Model file for the job. Use its own axes, mm. Coordinates: 2 decimals unless noted, no trailing zeros. Write each loop counter-clockwise with the first axis right and the second up, starting at its lowest first coordinate (ties: lowest second). Pieces come first, ordered by that corner, then holes. Notation, with made-up numbers: M 21.5,73 L 26.5,73 A15 ccw 26.5,91 Z; hole C 74,45 d3. An arc over 180 degrees is marked long. One line per question, with ' | ' between items. Start each with the question number.
(1) Flat gauge pin, fed straight in: pin 1 Ø9 at (x, z) = (-0.33, 0.13) entering from -Y. Where does the tip first touch, or does it go through?
(2) Cut at B-B (z = -41.5). Write the cut outline in (x, y), plus the area to 3 significant figures.
(3) Cut at C-C (y = -1.9). Count the separate pieces of the cut face and the enclosed holes in it, plus the area to 3 significant figures.
(4) Cut at A-A (x = 2). Write the cut outline in (y, z), plus the area to 3 significant figures.
(5) Wall check: probe 1 along X at (y, z) = (-2.6, -14); probe 2 along X at (y, z) = (-2.1, -58.5); probe 3 along Z at (x, y) = (22.5, -2.6). Give the ranges that are in metal, low to high.
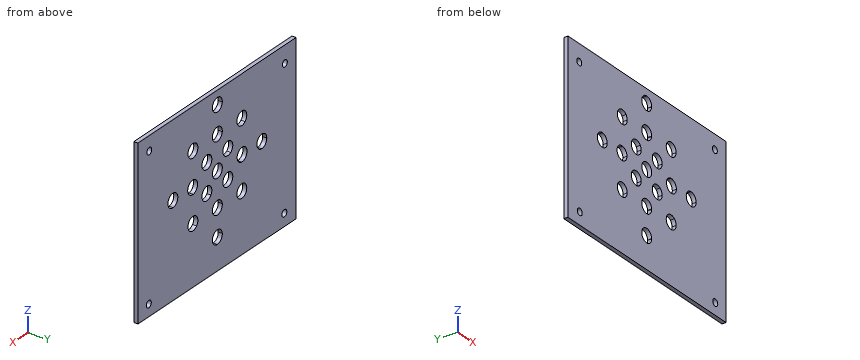
from build123d import *

# Parameters (mm, degrees)
F0_R     = 2.5
F0_R_2   = 5
F1_DEPTH = 3


with BuildPart() as f1:
    # F0 (on Front) → F1 (new body)
    with BuildSketch(Plane.XZ):
        Polygon((0, -68), (80, -68), (80, 55), (-80, 55.240198642), (-80, -68), align=None)
        with Locations((-68.1081116199, -58.9685998857)):
            Circle(F0_R, mode=Mode.SUBTRACT)
        with Locations((69.0506994724, -59.3423657119)):
            Circle(F0_R, mode=Mode.SUBTRACT)
        Polygon((49.6701618657, 0.1303526806), (49.6701618657, -49.8696473194), (-0.3298381532, -49.8696473194), (-50.3298381343, -49.8696473194), (-50.3298381343, 0.130352625), (-50.3298381343, 50.1303526806), (-0.3298380849, 50.1303526806), (49.6701618657, 50.1303526806), align=None, mode=Mode.SUBTRACT)
        with Locations((-68.6089098454, 42.6927655935)):
            Circle(F0_R, mode=Mode.SUBTRACT)
        with Locations((68.6089023948, 44.4455519319)):
            Circle(F0_R, mode=Mode.SUBTRACT)
        with BuildLine():
            ThreePointArc((-45.0520603566, -4.8619253071), (-32.1496432877, -31.6894524728), (-5.322116122, -44.5918695417))
            ThreePointArc((-5.322116122, -44.5918695417), (-0.3298381343, -39.8696473194), (4.6624398533, -44.5918695417))
            ThreePointArc((4.6624398533, -44.5918695417), (31.489967019, -31.6894524728), (44.3923840879, -4.8619253071))
            ThreePointArc((44.3923840879, -4.8619253071), (39.6701618657, 0.1303526806), (44.3923840879, 5.1226306682))
            ThreePointArc((44.3923840879, 5.1226306682), (31.489967019, 31.950157834), (4.6624398533, 44.8525749028))
            ThreePointArc((4.6624398533, 44.8525749028), (-0.3298381343, 40.1303526806), (-5.322116122, 44.8525749028))
            ThreePointArc((-5.322116122, 44.8525749028), (-32.1496432877, 31.950157834), (-45.0520603566, 5.1226306682))
            ThreePointArc((-45.0520603566, 5.1226306682), (-41.6974223481, 3.5662740353), (-40.3298381343, 0.1303526806))
            ThreePointArc((-40.3298381343, 0.1303526806), (-41.6974223481, -3.3055686741), (-45.0520603566, -4.8619253071))
        make_face()
        with BuildLine():
            ThreePointArc((27.6928642243, 21.1000487327), (32.8800593553, 11.1803621251), (34.6701618657, 0.1303526806))
            ThreePointArc((34.6701618657, 0.1303526806), (32.8800593553, -10.9196567639), (27.6928642243, -20.8393433716))
            ThreePointArc((27.6928642243, -20.8393433716), (28.9669661089, -22.5411058021), (29.4188992072, -24.618384661))
            ThreePointArc((29.4188992072, -24.618384661), (26.1660101872, -29.303211576), (20.6398579178, -27.8923496781))
            ThreePointArc((20.6398579178, -27.8923496781), (-0.3298381343, -34.8696473194), (-21.2995341865, -27.8923496781))
            ThreePointArc((-21.2995341865, -27.8923496781), (-28.6141093818, -28.1539185669), (-28.352540493, -20.8393433716))
            ThreePointArc((-28.352540493, -20.8393433716), (-35.3298381343, 0.1303526806), (-28.352540493, 21.1000487327))
            ThreePointArc((-28.352540493, 21.1000487327), (-28.6141093818, 28.414623928), (-21.2995341865, 28.1530550392))
            ThreePointArc((-21.2995341865, 28.1530550392), (-0.3298381343, 35.1303526806), (20.6398579178, 28.1530550392))
            ThreePointArc((20.6398579178, 28.1530550392), (26.1660101872, 29.5639169371), (29.4188992072, 24.8790900221))
            ThreePointArc((29.4188992072, 24.8790900221), (28.9669661089, 22.8018111633), (27.6928642243, 21.1000487327))
        make_face(mode=Mode.SUBTRACT)
        with BuildLine():
            ThreePointArc((27.6928642243, -20.8393433716), (32.8800593553, -10.9196567639), (34.6701618657, 0.1303526806))
            ThreePointArc((34.6701618657, 0.1303526806), (32.8800593553, 11.1803621251), (27.6928642243, 21.1000487327))
            ThreePointArc((27.6928642243, 21.1000487327), (20.8833653012, 21.3435561162), (20.6398579178, 28.1530550392))
            ThreePointArc((20.6398579178, 28.1530550392), (-0.3298381343, 35.1303526806), (-21.2995341865, 28.1530550392))
            ThreePointArc((-21.2995341865, 28.1530550392), (-20.3937485609, 26.6262010021), (-20.0785754759, 24.8790900221))
            ThreePointArc((-20.0785754759, 24.8790900221), (-23.0012966171, 20.3310231204), (-28.352540493, 21.1000487327))
            ThreePointArc((-28.352540493, 21.1000487327), (-35.3298381343, 0.1303526806), (-28.352540493, -20.8393433716))
            ThreePointArc((-28.352540493, -20.8393433716), (-23.0012966171, -20.0703177592), (-20.0785754759, -24.618384661))
            ThreePointArc((-20.0785754759, -24.618384661), (-20.3937485609, -26.365495641), (-21.2995341865, -27.8923496781))
            ThreePointArc((-21.2995341865, -27.8923496781), (-0.3298381343, -34.8696473194), (20.6398579178, -27.8923496781))
            ThreePointArc((20.6398579178, -27.8923496781), (20.8833653012, -21.082850755), (27.6928642243, -20.8393433716))
        make_face()
        with BuildLine():
            ThreePointArc((4.6450990512, 24.6303526806), (17.3478313953, 17.8080222102), (24.1701618657, 5.1052898661))
            ThreePointArc((24.1701618657, 5.1052898661), (28.0242638319, 3.8384519241), (29.6701618657, 0.1303526806))
            ThreePointArc((29.6701618657, 0.1303526806), (28.0242638319, -3.577746563), (24.1701618657, -4.844584505))
            ThreePointArc((24.1701618657, -4.844584505), (17.3478313953, -17.5473168491), (4.6450990512, -24.3696473194))
            ThreePointArc((4.6450990512, -24.3696473194), (4.6638922312, -24.6193334441), (4.6701618657, -24.8696473194))
            ThreePointArc((4.6701618657, -24.8696473194), (-0.5801520096, -29.863377685), (-5.3047753199, -24.3696473194))
            ThreePointArc((-5.3047753199, -24.3696473194), (-18.007507664, -17.5473168491), (-24.8298381343, -4.844584505))
            ThreePointArc((-24.8298381343, -4.844584505), (-30.3298381343, 0.1303526806), (-24.8298381343, 5.1052898661))
            ThreePointArc((-24.8298381343, 5.1052898661), (-18.007507664, 17.8080222102), (-5.3047753199, 24.6303526806))
            ThreePointArc((-5.3047753199, 24.6303526806), (-0.5801520096, 30.1240830461), (4.6701618657, 25.1303526806))
            ThreePointArc((4.6701618657, 25.1303526806), (4.6638922312, 24.8800388053), (4.6450990512, 24.6303526806))
        make_face(mode=Mode.SUBTRACT)
        with BuildLine():
            ThreePointArc((24.1701618657, -4.844584505), (19.6701618657, 0.1303526806), (24.1701618657, 5.1052898661))
            ThreePointArc((24.1701618657, 5.1052898661), (17.3478313953, 17.8080222102), (4.6450990512, 24.6303526806))
            ThreePointArc((4.6450990512, 24.6303526806), (-0.3298381343, 20.1303526806), (-5.3047753199, 24.6303526806))
            ThreePointArc((-5.3047753199, 24.6303526806), (-18.007507664, 17.8080222102), (-24.8298381343, 5.1052898661))
            ThreePointArc((-24.8298381343, 5.1052898661), (-21.6217388908, 3.4844546468), (-20.3298381343, 0.1303526806))
            ThreePointArc((-20.3298381343, 0.1303526806), (-21.6217388908, -3.2237492857), (-24.8298381343, -4.844584505))
            ThreePointArc((-24.8298381343, -4.844584505), (-18.007507664, -17.5473168491), (-5.3047753199, -24.3696473194))
            ThreePointArc((-5.3047753199, -24.3696473194), (-0.3298381343, -19.8696473194), (4.6450990512, -24.3696473194))
            ThreePointArc((4.6450990512, -24.3696473194), (17.3478313953, -17.5473168491), (24.1701618657, -4.844584505))
        make_face()
        with BuildLine():
            ThreePointArc((13.1735913764, 6.6616153035), (14.2912330073, 3.4806181431), (14.6701618657, 0.1303526806))
            ThreePointArc((14.6701618657, 0.1303526806), (14.2912330073, -3.219912782), (13.1735913764, -6.4009099423))
            ThreePointArc((13.1735913764, -6.4009099423), (14.7199684496, -8.1832312619), (15.2767635834, -10.4762490372))
            ThreePointArc((15.2767635834, -10.4762490372), (11.7971754562, -15.2394777465), (6.2014244886, -13.3730768301))
            ThreePointArc((6.2014244886, -13.3730768301), (-0.3298381343, -14.8696473194), (-6.8611007573, -13.3730768301))
            ThreePointArc((-6.8611007573, -13.3730768301), (-14.4719737581, -14.0117829432), (-13.833267645, -6.4009099423))
            ThreePointArc((-13.833267645, -6.4009099423), (-15.3298381343, 0.1303526806), (-13.833267645, 6.6616153035))
            ThreePointArc((-13.833267645, 6.6616153035), (-14.4719737581, 14.2724883043), (-6.8611007573, 13.6337821913))
            ThreePointArc((-6.8611007573, 13.6337821913), (-0.3298381343, 15.1303526806), (6.2014244886, 13.6337821913))
            ThreePointArc((6.2014244886, 13.6337821913), (11.7971754562, 15.5001831077), (15.2767635834, 10.7369543984))
            ThreePointArc((15.2767635834, 10.7369543984), (14.7199684496, 8.4439366231), (13.1735913764, 6.6616153035))
        make_face(mode=Mode.SUBTRACT)
        with BuildLine():
            Line((-0.3298381532, -49.8696473194), (49.6701618657, -49.8696473194))
            Line((49.6701618657, -49.8696473194), (49.6701618657, 0.1303526806))
            ThreePointArc((49.6701618657, 0.1303526806), (48.1060832203, -3.5020631057), (44.3923840879, -4.8619253071))
            ThreePointArc((44.3923840879, -4.8619253071), (31.489967019, -31.6894524728), (4.6624398533, -44.5918695417))
            ThreePointArc((4.6624398533, -44.5918695417), (4.6682309897, -44.7307047744), (4.6701618657, -44.8696473194))
            ThreePointArc((4.6701618657, -44.8696473194), (3.2056957649, -48.405181232), (-0.3298381532, -49.8696473194))
        make_face()
        with BuildLine():
            Line((-50.3298381343, -49.8696473194), (-0.3298381532, -49.8696473194))
            ThreePointArc((-0.3298381532, -49.8696473194), (-3.9622539271, -48.3055686673), (-5.322116122, -44.5918695417))
            ThreePointArc((-5.322116122, -44.5918695417), (-32.1496432877, -31.6894524728), (-45.0520603566, -4.8619253071))
            ThreePointArc((-45.0520603566, -4.8619253071), (-48.7657594688, -3.5020631248), (-50.3298381343, 0.130352625))
            Line((-50.3298381343, 0.130352625), (-50.3298381343, -49.8696473194))
        make_face()
        with BuildLine():
            ThreePointArc((44.3923840879, 5.1226306682), (48.1060832203, 3.7627684669), (49.6701618657, 0.1303526806))
            Line((49.6701618657, 0.1303526806), (49.6701618657, 50.1303526806))
            Line((49.6701618657, 50.1303526806), (-0.3298380849, 50.1303526806))
            ThreePointArc((-0.3298380849, 50.1303526806), (3.205695789, 48.665886569), (4.6701618657, 45.1303526806))
            ThreePointArc((4.6701618657, 45.1303526806), (4.6682309897, 44.9914101355), (4.6624398533, 44.8525749028))
            ThreePointArc((4.6624398533, 44.8525749028), (31.489967019, 31.950157834), (44.3923840879, 5.1226306682))
        make_face()
        with BuildLine():
            Line((-50.3298381343, 50.1303526806), (-50.3298381343, 0.130352625))
            ThreePointArc((-50.3298381343, 0.130352625), (-48.7657595092, 3.7627684478), (-45.0520603566, 5.1226306682))
            ThreePointArc((-45.0520603566, 5.1226306682), (-32.1496432877, 31.950157834), (-5.322116122, 44.8525749028))
            ThreePointArc((-5.322116122, 44.8525749028), (-3.9622539037, 48.5662740532), (-0.3298380849, 50.1303526806))
            Line((-0.3298380849, 50.1303526806), (-50.3298381343, 50.1303526806))
        make_face()
        with BuildLine():
            ThreePointArc((13.1735913764, -6.4009099423), (14.2912330073, -3.219912782), (14.6701618657, 0.1303526806))
            ThreePointArc((14.6701618657, 0.1303526806), (14.2912330073, 3.4806181431), (13.1735913764, 6.6616153035))
            ThreePointArc((13.1735913764, 6.6616153035), (6.7412296775, 7.2014204924), (6.2014244886, 13.6337821913))
            ThreePointArc((6.2014244886, 13.6337821913), (-0.3298381343, 15.1303526806), (-6.8611007573, 13.6337821913))
            ThreePointArc((-6.8611007573, 13.6337821913), (-6.1732111428, 12.2573662711), (-5.9364398521, 10.7369543984))
            ThreePointArc((-5.9364398521, 10.7369543984), (-8.6434220769, 6.2937495323), (-13.833267645, 6.6616153035))
            ThreePointArc((-13.833267645, 6.6616153035), (-15.3298381343, 0.1303526806), (-13.833267645, -6.4009099423))
            ThreePointArc((-13.833267645, -6.4009099423), (-8.6434220769, -6.0330441711), (-5.9364398521, -10.4762490372))
            ThreePointArc((-5.9364398521, -10.4762490372), (-6.1732111428, -11.99666091), (-6.8611007573, -13.3730768301))
            ThreePointArc((-6.8611007573, -13.3730768301), (-0.3298381343, -14.8696473194), (6.2014244886, -13.3730768301))
            ThreePointArc((6.2014244886, -13.3730768301), (6.7412296775, -6.9407151313), (13.1735913764, -6.4009099423))
        make_face()
        with Locations((-0.3298381343, 0.1303526806)):
            Circle(F0_R_2, mode=Mode.SUBTRACT)
    extrude(amount=F1_DEPTH)


solid = f1.part
Filled in:
1) pin 1: through
2) outline: M -80,-3 L -4.02,-3 L -4.02,0 L -80,0 Z; M 3.36,-3 L 80,-3 L 80,0 L 3.36,0 Z | area: 458 mm²
3) separate pieces: 1 | enclosed holes: 21 | area: 18,300 mm²
4) outline: M -3,-68 L 0,-68 L 0,-49.29 L -3,-49.29 Z; M -3,-40.45 L 0,-40.45 L 0,-29.29 L -3,-29.29 Z; M -3,-20.45 L 0,-20.45 L 0,-4.29 L -3,-4.29 Z; M -3,4.55 L 0,4.55 L 0,20.71 L -3,20.71 Z; M -3,29.55 L 0,29.55 L 0,40.71 L -3,40.71 Z; M -3,49.55 L 0,49.55 L 0,55.12 L -3,55.12 Z | area: 237 mm²
5) probe 1: -80 to -14.48, -7.39 to 6.73, 13.82 to 80 | probe 2: -80 to -70.56, -65.65 to 66.7, 71.4 to 80 | probe 3: -68 to -29.24, -20 to -4.37, 4.63 to 20.26, 29.5 to 55.09
